Geometry: final body of the model. Coordinates: model frame, mm. Coordinates: 2 decimals unless noted, no trailing zeros. Write each question's results on one line, items separated by ' | '. Start each with the question number.
Autodesk Inventor part; units mm, degrees
ref_plane "YZ Plane" through (0, 0, 0) normal (1, 0, 0) x (0, 1, 0)
ref_plane "XZ Plane" through (0, 0, 0) normal (0, 1, 0) x (-1, 0, 0)
ref_plane "XY Plane" through (0, 0, 0) normal (0, 0, 1) x (1, 0, 0)
sketch "Sketch8" plane through (0, 0, 0) normal (0, 0, 1) x (1, 0, 0)
  line L0 (-1260, 50) -> (1260, 50)
  line L1 (1260, 50) -> (1260, 0)
  line L2 (1260, 0) -> (-1260, 0)
  line L3 (-1260, 0) -> (-1260, 50)
  point P0 (0, 0)
  point P1 (0, 0)
  dimension "d37" = 50
  dimension "d38" = 2520
extrude "Plate5" add sketch "Sketch8" against normal blind 3
sketch "Sketch9" plane through (0, 0, 0) normal (0, 0, 1) x (1, 0, 0)
  line L0 (1260, 50) -> (-1260, 50)
  line L1 (-1011.6, 50) -> (-1008.4, 50)
  line L2 (-1008.4, 50) -> (-1008.4, 24)
  line L3 (-1008.4, 24) -> (-1011.6, 24)
  line L4 (-1011.6, 24) -> (-1011.6, 50)
  point P0 (0, 0)
  point P1 (-1008.4, 50)
  dimension "d40" = 248.4
  dimension "d41" = 3.2
  dimension "d42" = 26
extrude "Extrusion3" cut sketch "Sketch9" against normal through all
pattern_linear "Rectangular Pattern2" count 5 spacing 500 along (1, 0, 0) of "Extrusion3"
sketch "Sketch10" plane through (0, 0, -3) normal (0, 0, -1) x (-1, 0, 0)
  line L0 (-988.4, 50) -> (-988.4, 24)
  line L1 (-988.4, 24) -> (-991.6, 24)
  line L2 (-991.6, 24) -> (-991.6, 50)
  line L3 (-1260, 50) -> (-991.6, 50)
  line L4 (-1260, 0) -> (-1260, 50)
  line L5 (1260, 0) -> (-1260, 0)
  line L6 (1260, 50) -> (1260, 0)
  line L7 (1011.6, 50) -> (1260, 50)
  line L8 (1011.6, 50) -> (1011.6, 24)
  line L9 (1011.6, 24) -> (1008.4, 24)
  line L10 (1008.4, 24) -> (1008.4, 50)
  line L11 (511.6, 50) -> (1008.4, 50)
  line L12 (511.6, 50) -> (511.6, 24)
  line L13 (511.6, 24) -> (508.4, 24)
  line L14 (508.4, 24) -> (508.4, 50)
  line L15 (11.6, 50) -> (508.4, 50)
  line L16 (11.6, 50) -> (11.6, 24)
  line L17 (11.6, 24) -> (8.4, 24)
  line L18 (8.4, 24) -> (8.4, 50)
  line L19 (-488.4, 50) -> (8.4, 50)
  line L20 (-488.4, 50) -> (-488.4, 24)
  line L21 (-488.4, 24) -> (-491.6, 24)
  line L22 (-491.6, 24) -> (-491.6, 50)
  line L23 (-988.4, 50) -> (-491.6, 50)
  circle A0 centre (750, 50) radius 20
  line L24 (11.6, 50) -> (508.4, 50)
  circle A1 centre (-730, 50) radius 20
  point P0 (0, 0)
  point P1 (770, 50)
  point P2 (730, 50)
  point P3 (-710, 50)
  point P4 (-750, 50)
  dimension "d48" = 40
  dimension "d49" = 40
  dimension "d50" = 1480
  dimension "d51" = 530
extrude "Extrusion4" cut sketch "Sketch10" against normal through all contours L23 A1 | A0 L11 picked at (-735.7537, 42.481) picked at (744.2463, 42.481)
equation "\"d39\" = Thickness"
equation "\"BendReliefWidth\" = Thickness"
equation "\"BendReliefDepth\" = 0.5 * Thickness"
equation "\"CornerReliefSize\" = 4 * Thickness"
equation "\"MinimumRemnant\" = 2 * Thickness"
equation "\"TransitionRadius\" = BendRadius"
equation "\"JacobiRadiusSize\" = BendRadius"
equation "\"GapSize\" = Thickness"
properties part number "BSH 031 stringer floor" material "09g2s"
1) Section query A-A on y = 40.5. Count the separate pieces of the cut face and the enclosed holes in it, and give its area (3 significant figures).
2) Material intervals for line 1 (X direction, y = 26.5, z = -1.15), sorted ascending. Write a range as [from, to].
3) Pin query (flat end, axial travel): pin 1 Ø1.5 at (x, z) = (990.5, -2) entering from +Y. Return the tip coordinate at first contact, or that it passes through.
Returned:
1) separate pieces: 8 | enclosed holes: 0 | area: 7,300 mm²
2) line 1: x = [-1260, -1011.6], [-1008.4, -511.6], [-508.4, -11.6], [-8.4, 488.4], [491.6, 988.4], [991.6, 1260]
3) pin 1: stops at y = 24
